The listing builds one solid part. Answer for the finished solid, in the listing's coordinates (mm). Face numbers are marked on the shaded views. Give positions to 0.01 mm unless a question says otherwise; leave off trailing zeros. Loops run counter-clockwise (first coordinate to the right, second up) from the corner with the lowest first, then second, coordinate; pieces in that order, holes last. Notation, with made-up numbers: (-16.75, -23) - (13.25, -23) arc R19 cw to (13.25, 6) - close; hole circle Ø7 at (-32, 9). An arc over 180 degrees is marked (long way). One line per item, written item: value. Start each with the question number.
from build123d import *

# Parameters (mm, degrees)
SKETCH1_W           = 15
SKETCH1_H           = 34
BOSS_EXTRUDE1_DEPTH = 75
CUT_EXTRUDE5_DEPTH  = 15
CUT_EXTRUDE6_START  = -15
CUT_EXTRUDE6_DEPTH  = 10
SKETCH13_W          = 23
SKETCH13_H          = 4
BOSS_EXTRUDE4_DEPTH = 15
SKETCH14_R          = 1.85
CUT_EXTRUDE8_DEPTH  = 85.107074613
SKETCH15_W          = 9
SKETCH15_H          = 14
BOSS_EXTRUDE5_DEPTH = 10
CUT_EXTRUDE4_REACH  = 97.389
SKETCH5_R           = 1.9
SKETCH11_R          = 4.6
CUT_EXTRUDE7_DEPTH  = 10
SKETCH12_R          = 4.6
SKETCH12_R_2        = 3.1
BOSS_EXTRUDE3_DEPTH = 2
SKETCH20_W          = 40
SKETCH20_H          = 5
BOSS_EXTRUDE8_DEPTH = 15
SKETCH21_R          = 3.5
CUT_EXTRUDE11_DEPTH = 103.961157725
SKETCH22_R          = 1.95
CUT_EXTRUDE12_DEPTH = 167.595318061


with BuildPart() as part:
    # Sketch1 → Boss-Extrude1 (new body)
    with BuildSketch(Plane(origin=(0, 0, 0), x_dir=(1, 0, 0), z_dir=(0, 1, 0))):
        with Locations((7.5, 17)):
            Rectangle(SKETCH1_W, SKETCH1_H)
    extrude(amount=BOSS_EXTRUDE1_DEPTH)

    # Sketch2 → Cut-Extrude5 (cut)
    with BuildSketch(Plane(origin=(15, 0, 0), x_dir=(0, 0, -1), z_dir=(1, 0, 0))):
        Polygon((0, 75), (0, 65), (24, 75), align=None)
        Polygon((0, 0), (24, 0), (0, 10), align=None)
    extrude(amount=-CUT_EXTRUDE5_DEPTH, mode=Mode.SUBTRACT)

    # Sketch2<5> → Cut-Extrude6 (cut)
    with BuildSketch(Plane(origin=(15, 0, 0), x_dir=(0, 0, -1), z_dir=(1, 0, 0)).offset(CUT_EXTRUDE6_START)):
        Polygon((25, 5), (34, 5), (34, 70), (25, 70), (5, 61.666666667), (5, 13.333333333), align=None)
    extrude(amount=CUT_EXTRUDE6_DEPTH, mode=Mode.SUBTRACT)

    # Sketch13 → Boss-Extrude4 (add)
    with BuildSketch(Plane(origin=(15, 0, 0), x_dir=(0, 0, -1), z_dir=(1, 0, 0))):
        with Locations((45.5, 58)):
            Rectangle(SKETCH13_W, SKETCH13_H)
    extrude(amount=-BOSS_EXTRUDE4_DEPTH)

    # Sketch14 → Cut-Extrude8 (cut, through all)
    with BuildSketch(Plane(origin=(0, 60, 0), x_dir=(1, 0, 0), z_dir=(0, 1, 0))):
        with Locations(Location((6, 39, 0), (0, 0, 270))):
            Circle(SKETCH14_R)
        with Locations(Location((6, 52, 0), (0, 0, 270))):
            Circle(SKETCH14_R)
    extrude(amount=-CUT_EXTRUDE8_DEPTH, mode=Mode.SUBTRACT)

    # Sketch15 → Boss-Extrude5 (add)
    with BuildSketch(Plane.ZY.offset(-10)):
        with Locations((-29.5, 63)):
            Rectangle(SKETCH15_W, SKETCH15_H)
    extrude(amount=BOSS_EXTRUDE5_DEPTH)

    # Cut-Extrude4: up to this face of the body (flat: up to its plane)
    cut_extrude4_end = Plane(part.part.faces().sort_by_distance((7.5, 0, -29))[0])
    # Sketch5 → Cut-Extrude4 (cut, up to the picked face)
    with BuildSketch(Plane(origin=(0, 75, 0), x_dir=(1, 0, 0), z_dir=(0, 1, 0)), mode=Mode.PRIVATE) as cut_extrude4_sk1:
        with Locations(Location((5, 30.25, 0), (0, 0, 270))):
            Circle(SKETCH5_R)
    cut_extrude4_tool1 = split(extrude(cut_extrude4_sk1.sketch, amount=-CUT_EXTRUDE4_REACH, mode=Mode.PRIVATE), bisect_by=cut_extrude4_end, keep=Keep.BOTH, mode=Mode.PRIVATE)
    add(cut_extrude4_tool1.solids().sort_by(Axis((5, 75, -30.25), (0, -1, 0)))[0], mode=Mode.SUBTRACT)

    # Sketch11 → Cut-Extrude7 (cut)
    with BuildSketch(Plane(origin=(15, 0, 0), x_dir=(0, 0, -1), z_dir=(1, 0, 0))):
        with Locations((13.2, 31)):
            Circle(SKETCH11_R)
    extrude(amount=-CUT_EXTRUDE7_DEPTH, mode=Mode.SUBTRACT)

    # Sketch12 → Boss-Extrude3 (add)
    with BuildSketch(Plane(origin=(15, 0, 0), x_dir=(0, 0, -1), z_dir=(1, 0, 0))):
        with Locations((13.2, 31)):
            Circle(SKETCH12_R)
        with Locations((13.2, 31)):
            Circle(SKETCH12_R_2, mode=Mode.SUBTRACT)
    extrude(amount=-BOSS_EXTRUDE3_DEPTH)

    # Sketch20 → Boss-Extrude8 (add)
    with BuildSketch(Plane.ZY):
        with Locations((-54, 2.5)):
            Rectangle(SKETCH20_W, SKETCH20_H)
    extrude(amount=-BOSS_EXTRUDE8_DEPTH)

    # Sketch21 → Cut-Extrude11 (cut, through all)
    with BuildSketch(Plane(origin=(0, 5, 0), x_dir=(1, 0, 0), z_dir=(0, 1, 0))):
        with Locations((0, 49.5)):
            Circle(SKETCH21_R)
    extrude(amount=-CUT_EXTRUDE11_DEPTH, mode=Mode.SUBTRACT)

    # Mirror3: part across plane


with BuildPart() as part_1:
    add(part.part)
    add(part.part.mirror(Plane(origin=(55.311288741, 0, -74), x_dir=(1, 0, 0), z_dir=(0, 0, -1))))

    # Sketch22 → Cut-Extrude12 (cut, through all)
    with BuildSketch(Plane.XY):
        with Locations((6, 27.5)):
            Circle(SKETCH22_R)
    extrude(amount=-CUT_EXTRUDE12_DEPTH, mode=Mode.SUBTRACT)


solid = part_1.part
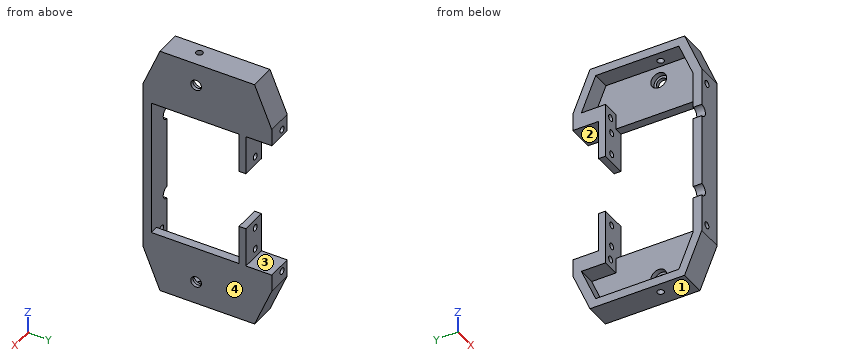
1. A cutting plane is placed at B-B (y = 21.5). Determine the outline of the cut face in (x, z), plus the area to 3 significant figures.
2. A cutting plane is placed at C-C (z = -109). Determine the outline of the cut face in (x, y).
3. A cutting plane is placed at D-D (z = -13.2). Determine the outline of the cut face in (x, y), plus the area to 3 significant figures.
4. Find the intervals of material crossed by L1, parallel to X at y = 58.8, z = -109; L2, parallel to Z at x = 6, y = 23; L3, parallel to Y at x = 3, z = -30, in increasing order. Write a range as [from, to].
5. Determine the mould class of the marked faces 1, 2, 3 and 4 for opening direction Z: released by +Z, released by -Z, zero draft, split by the parting line, or undercut.
6. A cutting plane is placed at A-A (y = 63). Determine the outline of the cut face in (x, z).
7. Flat-ended cylindrical pins translate along their axes: pin 1 (7.5 mm diameter, centred on y = 31, z = -134.8, fed in from +X); pin 2 (6 mm diameter, centred on y = 14.5, z = -16, fed in from -X); pin 3 (3.5 mm diameter, centred on x = 5, z = -117.75, fed in from +Y); pin 4 (7.5 mm diameter, centred on x = 8.5, z = -53, fed in from +Y). Find the tip coordinate at first contact, or state that the pin passes through.
Results below:
1. outline: (0, -148) - (15, -148) - (15, -114) - (10, -114) - (10, -143) - (0, -143) - close; (0, -5) - (10, -5) - (10, -34) - (15, -34) - (15, 0) - (0, 0) - close
1. area: 440 mm^2
2. outline: (0, 0) - (15, 0) - (15, 5) - (0, 5) - close; (0, 56) - (4.15, 56) - (4.15, 60) - (0, 60) - close; (7.85, 56) - (15, 56) - (15, 60) - (7.85, 60) - close
3. outline: (0, 4.5) - (15, 4.5) - (15, 27.9) - (13, 27.9) - (13, 26.4) - (10, 26.4) - (10, 9.92) - (0, 9.92) - close; (0, 65.08) - (10, 65.08) - (10, 35.6) - (13, 35.6) - (13, 34.1) - (15, 34.1) - (15, 70.5) - (0, 70.5) - close
3. area: 398 mm^2
4. L1: x = [0, 4.15], [7.85, 15]
4. L2: z = [-148, -143], [-5, 0]
4. L3: y = [0, 5], [56, 75]
5. face 1: released by -Z
5. face 2: undercut
5. face 3: undercut
5. face 4: zero draft
6. outline: (0, -148) - (15, -148) - (15, -114) - (0, -114) - (0, -123) - (10, -123) - (10, -139.8) - (0, -139.8) - close; (0, -34) - (15, -34) - (15, 0) - (0, 0) - (0, -8.2) - (10, -8.2) - (10, -25) - (0, -25) - close; hole circle Ø3.8 at (5, -117.75); hole circle Ø3.8 at (5, -30.25)
7. pin 1: stops at x = 15
7. pin 2: stops at x = 10
7. pin 3: passes through
7. pin 4: stops at y = 60
